Part model, mm, in its own coordinate system. Face numbers are marked on the shaded views. A direction names the side the tool comes from. Coordinates: 2 decimals unless noted, no trailing zeros. Loops run counter-clockwise (first coordinate to the right, second up) from the corner with the lowest first, then second, coordinate; pieces in that order, holes last. Notation, with made-up numbers: (16, -35) -> (48, -35) arc R17 ccw to (48, -14) -> close; hole circle Ø1 at (85, -22.75). An arc over 180 degrees is marked (long way). Use one line per item in the form item = value. Start each with the question number.
(1) Mould opens along X. For the marked faces 3, 4, 5 and 6 say: +X half, -X half, draft (parallel to the pull), parting line (faces both ways), or undercut.
(2) 3-axis set-ups, long thin cutter, end or side, ignore diameter. For the marked faces 1 and 2: which of +Z, -Z, +X, -X, +Y, -Y reach the whole face in a straight line?
(3) Band-saw the part on A-A on y = -3.5. Give the cut face in (x, z).
(4) Band-saw the part on C-C on z = 16.5. Give the cut face in (x, y), then the cut area to 3 significant figures.
(5) Band-saw the part on B-B on x = 34. Give the cut face in (y, z).
(6) Drill centre lines: L1, parallel to X at y = -7, z = 4.25; L2, parallel to Z at x = 40, y = -3; L3, parallel to Z at x = -7, y = -13. Where is each one in solid material? Low to high. Write a range as [from, to].
(7) Pin check, flat tips, straight feed: P1, Ø2.5, axis at x = 1, y = -11.5, coming from the +Z side; P2, Ø8, axis at x = -25.5, y = -8, coming from the +Z side; P3, Ø3.5, axis at x = -0.06, z = 6, coming from the -Y side; P4, Ø10, axis at x = 6, z = 11.5, coming from the -Y side. Stop position of each tip, or through.
```python
from build123d import *

# Parameters (mm, degrees)
F1_DEPTH = 19
F0_W     = 103
F0_H     = 9
F2_DEPTH = 2
F4_DEPTH = 120
F5_R     = 2.1
F6_DEPTH = 4.2


with BuildPart() as f1:
    # F0 (on Top) → F1 (new body)
    with BuildSketch(Plane.XY):
        Polygon((-52, -14), (-52, -5), (51, -5), (51, -14), (56, -14), (56, 0), (47.60337, 0), (45.10337, -2.5), (42.60337, 0), (17.60337, 0), (15.10337, -2.5), (12.60337, 0), (-12.39663, 0), (-14.89663, -2.5), (-17.39663, 0), (-42.39663, 0), (-44.89663, -2.5), (-47.39663, 0), (-57, 0), (-57, -14), align=None)
    extrude(amount=F1_DEPTH)

    # F0 (on Top) → F2 (join)
    with BuildSketch(Plane.XY):
        with Locations((-0.5, -9.5)):
            Rectangle(F0_W, F0_H)
    extrude(amount=F2_DEPTH)

    # F3 (on face) → F4 (cut)
    with BuildSketch(Plane.YZ.offset(56)):
        Polygon((0, 8), (0, 13), (-2.5, 10.5), align=None)
        Polygon((1.035534, 6.964466), (1.035534, 14.035534), (0, 13), (0, 8), align=None)
    extrude(amount=-F4_DEPTH, mode=Mode.SUBTRACT)

    # F5 (on face) → F6 (cut)
    with BuildSketch(Plane.XZ.offset(5)):
        with Locations((-40.057622, 6)):
            Circle(F5_R)
        with Locations((-0.057622, 6)):
            Circle(F5_R)
        with Locations((39.942378, 6)):
            Circle(F5_R)
    extrude(amount=-F6_DEPTH, mode=Mode.SUBTRACT)


solid = f1.part
```
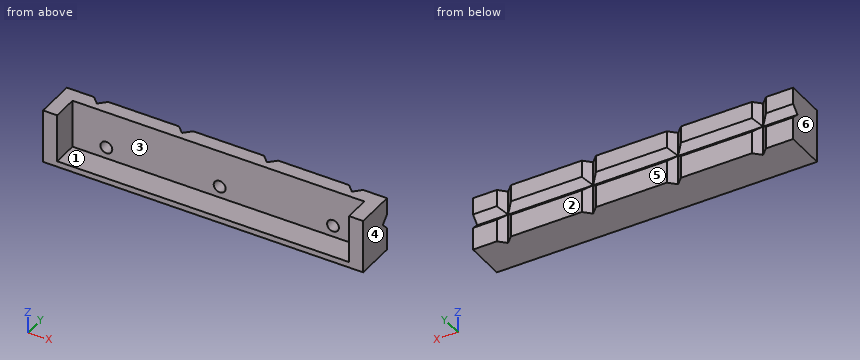
A:
q1.face_3 = undercut
q1.face_4 = +X half
q1.face_5 = draft
q1.face_6 = -X half
q2.face_1 = +Z, -Y
q2.face_2 = +Z, -Z, +X, -X, +Y
q3.outline = (-57, 0) -> (56, 0) -> (56, 19) -> (-57, 19) -> close; hole circle Ø4.2 at (-40.06, 6); hole circle Ø4.2 at (-0.06, 6); hole circle Ø4.2 at (39.94, 6)
q4.outline = (-57, -14) -> (-52, -14) -> (-52, -5) -> (51, -5) -> (51, -14) -> (56, -14) -> (56, 0) -> (47.6, 0) -> (45.1, -2.5) -> (42.6, 0) -> (17.6, 0) -> (15.1, -2.5) -> (12.6, 0) -> (-12.4, 0) -> (-14.9, -2.5) -> (-17.4, 0) -> (-42.4, 0) -> (-44.9, -2.5) -> (-47.4, 0) -> (-57, 0) -> close
q4.area = 630 mm²
q5.outline = (-14, 0) -> (0, 0) -> (0, 8) -> (-2.5, 10.5) -> (0, 13) -> (0, 19) -> (-5, 19) -> (-5, 2) -> (-14, 2) -> close
q6.L1 = [-57, -52], [51, 56]
q6.L2 = [0, 3.9], [8.1, 19]
q6.L3 = [0, 2]
q7.P1 = 2
q7.P2 = 19
q7.P3 = -0.8
q7.P4 = -5
